Print and shaded views of the part. All mm, measured from the part's lowest x, y and z. A direction names the side the tool comes from. Give positions to 0.01 mm unless a question says otherwise; leave off trailing zeros. Loops run counter-clockwise (first coordinate to the right, second up) from the corner with the lowest first, then second, coordinate; pieces in that order, holes last. Notation, with made-up numbers: M 81,-23 L 130,-23 A28 ccw 130,1 Z; hole C 42.25,-40 d8. An arc over 180 degrees is marked long. Put each result on its own line as item: value. Start each with the question number.
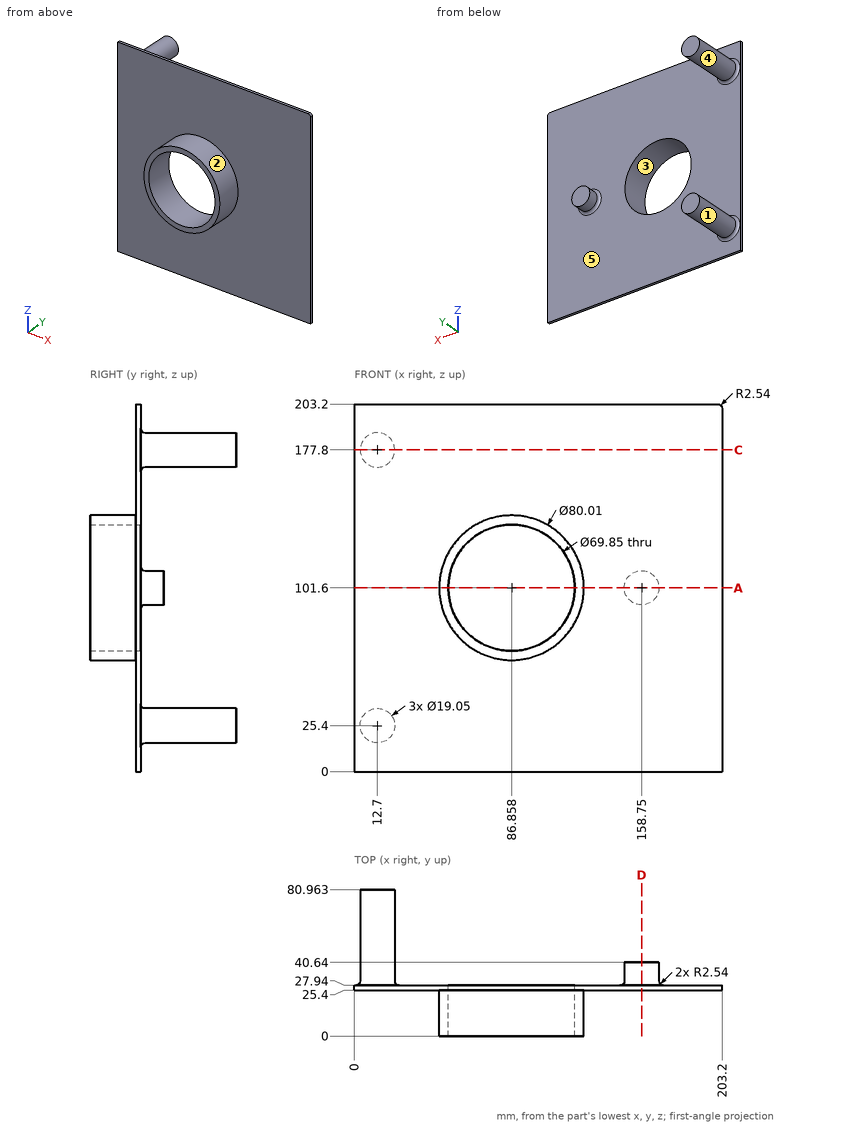
1) Band-saw the part on A-A on z = 101.6. Give the cut face in (x, y) (1 decimal).
2) Band-saw the part on D-D on x = 158.75. Give the cut face in (y, z) (1 decimal).
3) Which spindle directions (+Z, -Z, +X, -X, +Y, -Y) get a long thin tool onto all of the face, cutting with end or side? Do the marked faces 1 and 2. Say none if no direction does.
4) Band-saw the part on C-C on z = 177.8. Give the cut face in (x, y) (1 decimal), then the cut area to 3 significant figures.
5) Wall check: L1, parallel to X at y = 16.5, z = 101; L2, parallel to Y at x = 44, z = 42; L3, parallel to Z at x = 61, y = 5.5 (1 decimal). Give the ranges that are in metal, low to high.
6) Pin check, flat tips, straight feed: pin 1 Ø10 at (x, z) = (97.5, 51) entering from -Y; pin 2 Ø3 at (x, y) = (96, 13) entering from -Z; pin 3 Ø10 at (y, z) = (14, 108.5) entering from -X. Stop position of each tip, or through.
7) Mould opens along X. For the marked faces 3, 4 and 5 say: +X half, -X half, draft (parallel to the pull), parting line (faces both ways), or undercut.
Evaluation:
1. outline: M 0,25.4 L 46.9,25.4 L 46.9,0 L 51.9,0 L 51.9,27.9 L 0,27.9 Z; M 121.8,0 L 126.9,0 L 126.9,25.4 L 203.2,25.4 L 203.2,27.9 L 170.8,27.9 A2.5 cw 168.3,30.5 L 168.3,40.6 L 149.2,40.6 L 149.2,30.5 A2.5 cw 146.7,27.9 L 121.8,27.9 Z
2. outline: M 25.4,0 L 27.9,0 L 27.9,89.5 A2.5 cw 30.5,92.1 L 40.6,92.1 L 40.6,111.1 L 30.5,111.1 A2.5 cw 27.9,113.7 L 27.9,203.2 L 25.4,203.2 Z
3. face 1: +Y
3. face 2: -Y
4. outline: M 0,25.4 L 203.2,25.4 L 203.2,27.9 L 24.8,27.9 A2.5 cw 22.2,30.5 L 22.2,81 L 3.2,81 L 3.2,30.5 A2.5 cw 0.6,27.9 L 0,27.9 Z
4. area: 1,530 mm2
5. L1: 46.86 to 51.94, 121.78 to 126.86
5. L2: 25.4 to 27.94
5. L3: 71.1 to 78.1, 125.1 to 132.1
6. pin 1: y = 25.4
6. pin 2: z = 62.33
6. pin 3: x = 46.9
7. face 3: undercut
7. face 4: parting line
7. face 5: draft
